Source: CAD feature listing. Evaluate the final solid. Frame: model axes, mm. Face numbers are marked on the shaded views. Round coordinates to 2 decimals unless told otherwise and drop trailing zeros. Loops run counter-clockwise (first coordinate to the right, second up) from the corner with the lowest first, then second, coordinate; pieces in that order, holes last.
Item 1: Section query D-D on x = 15.5. Return loops of the section in (y, z), then the cut area to 3 significant figures.
Item 2: Ray query, L1, parallel to X at y = -4, z = 19; L2, parallel to X at y = -6.5, z = 22; L3, parallel to Z at x = 17.78, y = -9.5. Return the intervals inside material, ascending.
Item 3: Pull-direction query (Z, two-part tool) for the marked faces 1, 2, 3 and 4; classes: released by +Z, released by -Z, zero draft, split by the parting line, or undercut.
Item 4: Section query B-B on z = 19.05. Return loops of the section in (x, y).
Item 5: Section query A-A on x = 66.04. Return loops of the section in (y, z).
Item 6: Section query C-C on y = -16.5. Return loops of the section in (x, z).
```python
from build123d import *

# Parameters (mm, degrees)
F0_W     = 83.82
F0_H     = 38.1
F1_DEPTH = 25.4
F2_R     = 5.08
F3_R     = 6.35
F4_DEPTH = 25.4
F5_SIZE  = 1.27


with BuildPart() as f1:
    # F0 (on Front) → F1 (new body)
    with BuildSketch(Plane.XZ):
        with Locations((41.91, 19.05)):
            Rectangle(F0_W, F0_H)
    extrude(amount=F1_DEPTH)

    # F2
    f2_edges = [f1.edges().sort_by_distance(p)[0] for p in [
        (83.82, -12.7, 38.1),
        (0, -12.7, 38.1),
        (83.82, -12.7, 0),
        (0, -12.7, 0),
    ]]
    fillet(f2_edges, radius=F2_R)

    # F3 (on face) → F4 (cut, through all)
    with BuildSketch(Plane.XZ.offset(25.4)):
        with Locations((17.78, 19.05)):
            Circle(F3_R)
        with Locations((66.04, 19.05)):
            Circle(F3_R)
    extrude(amount=-F4_DEPTH, mode=Mode.SUBTRACT)

    # F5
    f5_edges = [f1.edges().sort_by_distance(p)[0] for p in [
        (41.91, -25.4, 38.1),
        (41.91, 0, 38.1),
    ]]
    chamfer(f5_edges, length=F5_SIZE)


solid = f1.part
```
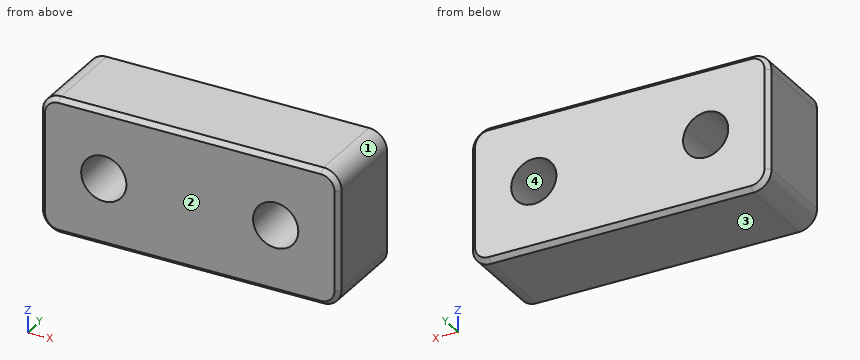
Data:
1. outline: (-25.4, 1.27) - (-24.13, 0) - (-1.27, 0) - (0, 1.27) - (0, 13.12) - (-25.4, 13.12) - close; (-25.4, 24.98) - (0, 24.98) - (0, 36.83) - (-1.27, 38.1) - (-24.13, 38.1) - (-25.4, 36.83) - close
1. area: 663 mm2
2. L1: x = 0 to 11.43, 24.13 to 59.69, 72.39 to 83.82
2. L2: x = 0 to 12.16, 23.4 to 60.42, 71.66 to 83.82
2. L3: z = 0 to 12.7, 25.4 to 38.1
3. face 1: released by +Z
3. face 2: zero draft
3. face 3: released by -Z
3. face 4: undercut
4. outline: (0, -24.13) - (1.27, -25.4) - (11.43, -25.4) - (11.43, 0) - (1.27, 0) - (0, -1.27) - close; (24.13, -25.4) - (59.69, -25.4) - (59.69, 0) - (24.13, 0) - close; (72.39, -25.4) - (82.55, -25.4) - (83.82, -24.13) - (83.82, -1.27) - (82.55, 0) - (72.39, 0) - close
5. outline: (-25.4, 1.27) - (-24.13, 0) - (-1.27, 0) - (0, 1.27) - (0, 12.7) - (-25.4, 12.7) - close; (-25.4, 25.4) - (0, 25.4) - (0, 36.83) - (-1.27, 38.1) - (-24.13, 38.1) - (-25.4, 36.83) - close
6. outline: (0, 5.08) arc R5.08 ccw to (5.08, 0) - (78.74, 0) arc R5.08 ccw to (83.82, 5.08) - (83.82, 33.02) arc R5.08 ccw to (78.74, 38.1) - (5.08, 38.1) arc R5.08 ccw to (0, 33.02) - close; hole circle Ø12.7 at (17.78, 19.05); hole circle Ø12.7 at (66.04, 19.05)
